Verification items for the finished model (mm, model axes). Face numbers are marked on the shaded views. Coordinates: 2 decimals unless noted, no trailing zeros. Write each loop counter-clockwise with the first axis right and the second up, starting at its lowest first coordinate (ties: lowest second). Pieces come first, ordered by that corner, then holes. Notation, with made-up numbers: M -13,61 L 37,61 A20 cw 37,71 Z; hole C -31,-2.5 d6. An arc over 180 degrees is marked long. Answer in a Markdown table with one row per item.
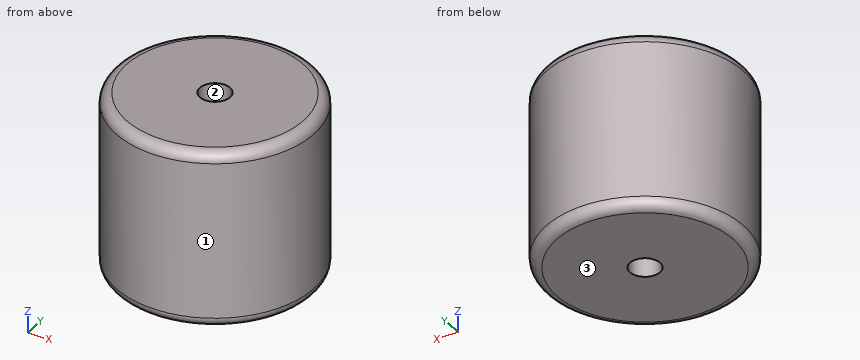
from build123d import *

# Parameters (mm, degrees)
SKETCH1_R           = 9.5
BOSS_EXTRUDE1_DEPTH = 17
FILLET1_R           = 1
SKETCH2_R           = 1.45
CUT_EXTRUDE1_DEPTH  = 17


with BuildPart() as part:
    # Sketch1 → Boss-Extrude1 (new body)
    with BuildSketch(Plane.XY):
        Circle(SKETCH1_R)
    extrude(amount=BOSS_EXTRUDE1_DEPTH)

    # Fillet1
    fillet1_edges = [part.edges().sort_by_distance(p)[0] for p in [
        (-9.5, 0, 0),
        (-9.5, 0, 17),
    ]]
    fillet(fillet1_edges, radius=FILLET1_R)

    # Sketch2 → Cut-Extrude1 (cut)
    with BuildSketch(Plane.XY.offset(17)):
        Circle(SKETCH2_R)
    extrude(amount=-CUT_EXTRUDE1_DEPTH, mode=Mode.SUBTRACT)


solid = part.part
1) Thickness scan on L1, parallel to Y at x = 0, z = 13.5; L2, parallel to X at y = -1.25, z = 3.75; L3, parallel to Y at x = 4.25, z = 8.75. Record the ranges inside material, lowest first. Write a range as [from, to].
Response values:
| item | result |
|---|---|
| L1 | y = [-9.5, -1.45], [1.45, 9.5] |
| L2 | x = [-9.42, -0.73], [0.73, 9.42] |
| L3 | y = [-8.5, 8.5] |
2) Depth check by flat-ended pin: pin 1 (10 mm diameter, centred on y = 6.5, z = 7.5, fed in from +X); pin 2 (1 mm diameter, centred on y = 1, z = 4, fed in from -X); pin 3 (4 mm diameter, centred on x = 5, z = 6.5, fed in from +Y). Enter the tip coordinate at first touch or a pass-through.
Response values:
| item | result |
|---|---|
| pin 1 | stops at x = 9.38 |
| pin 2 | stops at x = -9.49 |
| pin 3 | stops at y = 9.01 |
3) Release check for a two-part mould opening along X. For the marked faces 1, 2 and 3 record: +X half, -X half, draft (parallel to the pull), parting line (faces both ways), or undercut.
Response values:
| item | result |
|---|---|
| face 1 | parting line |
| face 2 | undercut |
| face 3 | draft |
4) Sectioned sample at A-A (y = 0). Record the cut outline in (x, z).
Response values:
| item | result |
|---|---|
| outline | M -9.5,1 A1 ccw -8.5,0 L -1.45,0 L -1.45,17 L -8.5,17 A1 ccw -9.5,16 Z; M 1.45,0 L 8.5,0 A1 ccw 9.5,1 L 9.5,16 A1 ccw 8.5,17 L 1.45,17 Z |
5) Sectioned sample at C-C (z = 5.25). Record the cut outline in (x, y).
Response values:
| item | result |
|---|---|
| outline | C 0,0 d19; hole C 0,0 d2.9 |
